from build123d import *

# Parameters (mm, degrees)
F1_DEPTH = 25.4
F3_DEPTH = 25.4


with BuildPart() as f1:
    # F0 (on Top) → F1 (new body)
    with BuildSketch(Plane.XY):
        Polygon((22.881487, 0), (0, 0), (0, -34.925), (45.762975, -61.346266), (77.856142, -61.346266), (123.369409, -35.069169), (123.369409, 0), (100.435721, 0), (76.2, 0), (45.762975, 0), align=None)
    extrude(amount=F1_DEPTH)

    # F2 (on face) → F3 (join)
    with BuildSketch(Plane.XY.offset(25.4)):
        Polygon((101.144409, 0), (22.225, 0), (22.225, -47.75661), (45.762975, -61.346266), (77.856142, -61.346266), (101.394116, -47.75661), align=None)
    extrude(amount=F3_DEPTH)


solid = f1.part
Source: CAD feature listing. Evaluate the final solid. Frame: model axes, mm. A direction names the side the tool comes from. Give positions to 0.01 mm unless a question says otherwise; leave off trailing zeros. Loops run counter-clockwise (first coordinate to the right, second up) from the corner with the lowest first, then second, coordinate; pieces in that order, holes last. Notation, with made-up numbers: (-11, -37.5) -> (32, -37.5) arc R25 cw to (32, -14.5) -> close; hole circle Ø7 at (62.5, 70). An arc over 180 degrees is marked (long way). Use a Markdown table: item, result. Add a question column.
1) Reachability of faces 1 (the face through (63, 0, 19)), 2 (the face through (22.225, -24, 38)) from +Z, -Z, +X, -X, +Y, -Y: full face, straight path, thin tool, end or side. Return the list, or none.
2) Line query: line 1 along X through (y, z) = (-43, 48) (3 decimals); line 2 along Z through (x, y) = (11.5, -34); line 3 along Y through (x, z) = (42, 8). Output: solid intervals per line, ascending. Write a range as [from, to].
3) Section query C-C, the plane x = 37. Return the cut outline in (y, z), then the cut area to 3 significant figures.
4) First-contact query: pin 1 (4 mm diameter, centred on x = 30.5, z = 11.5, fed in from -Y); pin 2 (6.5 mm diameter, centred on x = 11.5, y = -29, fed in from +Z); pin 3 (2 mm diameter, centred on y = -37, z = 6.5, fed in from +X). Flat tips, straight axial feed; report the tip coordinate or a pass-through.
5) Section query B-B, the plane y = -39. Return the cut outline in (x, z) (3 decimals).
6) Section query D-D, the plane y = -29. Return the cut outline in (x, z) (3 decimals).
7) Section query A-A, the plane z = 40. Return the cut outline in (x, y) (3 decimals).
Numbers:
| question | item | result |
|---|---|---|
| 1 | face 1 | +Z, -Z, +X, -X, +Y |
| 1 | face 2 | +Z, -X, +Y, -Y |
| 2 | line 1 | x = [22.225, 101.369] |
| 2 | line 2 | z = [0, 25.4] |
| 2 | line 3 | y = [-59.17, 0] |
| 3 | outline | (-56.29, 0) -> (0, 0) -> (0, 50.8) -> (-56.29, 50.8) -> close |
| 3 | area | 2,860 mm2 |
| 4 | pin 1 | stops at y = -53.69 |
| 4 | pin 2 | stops at z = 25.4 |
| 4 | pin 3 | stops at x = 121.76 |
| 5 | outline | (7.058, 0) -> (116.561, 0) -> (116.561, 25.4) -> (101.348, 25.4) -> (101.348, 50.8) -> (22.225, 50.8) -> (22.225, 25.4) -> (7.058, 25.4) -> close |
| 6 | outline | (0, 0) -> (123.369, 0) -> (123.369, 25.4) -> (101.296, 25.4) -> (101.296, 50.8) -> (22.225, 50.8) -> (22.225, 25.4) -> (0, 25.4) -> close |
| 7 | outline | (22.225, -47.757) -> (45.763, -61.346) -> (77.856, -61.346) -> (101.394, -47.757) -> (101.144, 0) -> (22.225, 0) -> close |
